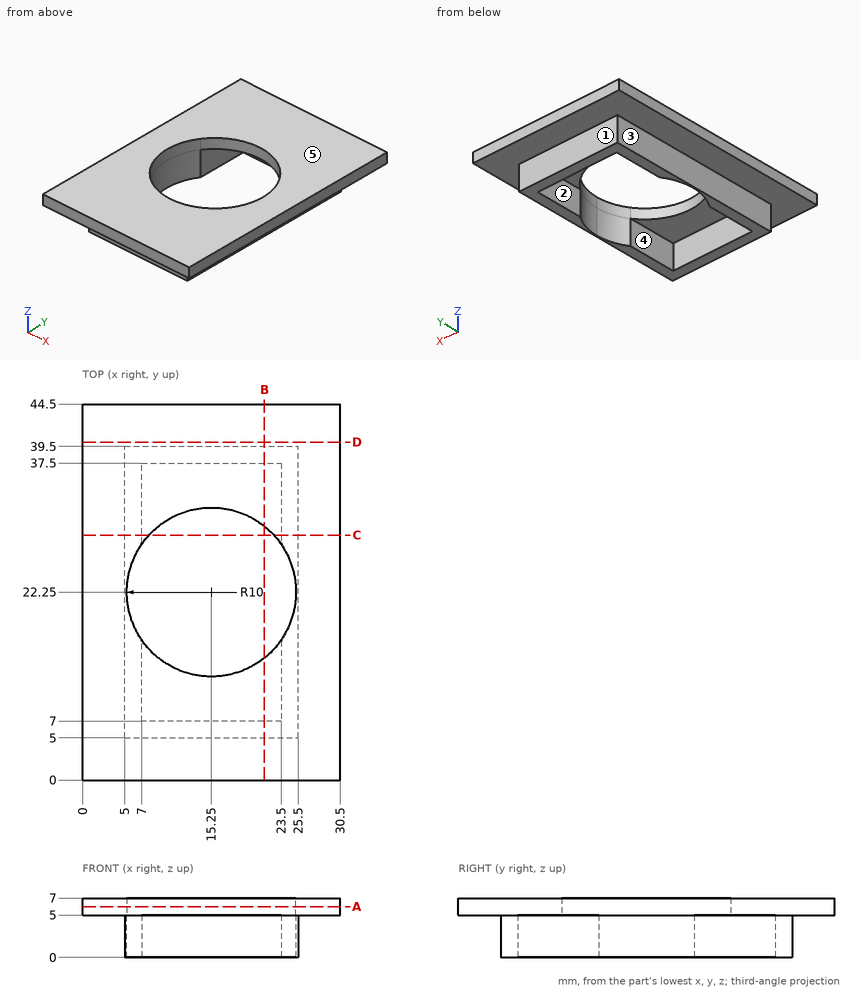
Here's the drawing with two shaded views (mm, measured from the low corner). I have some questions. A direction names the side the tool comes from. Round coordinates to 2 decimals unless told otherwise and drop trailing zeros. Order: outer loops, then holes, each group sorted by start corner. A loop starts at its lowest first (then second) coordinate and runs counter-clockwise, first axis right, second up. Notation, with made-up numbers: M 63.25,14 L 110.25,14 A35 ccw 110.25,47 Z; hole C 38.5,26 d9. An arc over 180 degrees is marked long. Answer in a Markdown table with one row per item.
Item 1: Imagine slicing it at A-A, the plane z = 6. Write out the boundary of the cut face in (x, y).
A:
| item | result |
|---|---|
| outline | M 0,0 L 30.5,0 L 30.5,44.5 L 0,44.5 Z; hole C 15.25,22.25 d20 |
Item 2: Imagine slicing it at D-D, the plane y = 40. Write out the boundary of the cut face in (x, z), and give its area (3 significant figures).
A:
| item | result |
|---|---|
| outline | M 0,5 L 30.5,5 L 30.5,7 L 0,7 Z |
| area | 61.0 mm2 |
Item 3: I'm going to push flat-ended pins straight in: pin 1 (10.5 mm diameter, centred on x = 17, y = 13.5, fed in from -Z); pin 2 (1.5 mm diameter, centred on x = 12.5, z = 2.5, fed in from -Y); pin 3 (1.5 mm diameter, centred on y = 11.5, z = 2, fed in from +X); pin 4 (4 mm diameter, centred on x = 23.5, z = 4.5, fed in from -Y). Where does each tip first touch, or does it pass through?
A:
| item | result |
|---|---|
| pin 1 | stops at z = 5 |
| pin 2 | stops at y = 5 |
| pin 3 | stops at x = 25.5 |
| pin 4 | stops at y = 0 |
Item 4: Imagine slicing it at B-B, the plane x = 21.5. Write out the boundary of the cut face in (y, z), and give its area (3 significant figures).
A:
| item | result |
|---|---|
| outline | M 0,5 L 5,5 L 5,0 L 7,0 L 7,5 L 14.44,5 L 14.44,7 L 0,7 Z; M 30.06,5 L 37.5,5 L 37.5,0 L 39.5,0 L 39.5,5 L 44.5,5 L 44.5,7 L 30.06,7 Z |
| area | 77.8 mm2 |
Item 5: If I drill on L1, parallel to X at y = 35, z = 1.5; L2, parallel to Y at x = 10.5, z = 0.75; L3, parallel to Y at x = 15.5, z = 5.25, over which ranges is the centre line in solid material (lowest first)? Write a range as from..to.
A:
| item | result |
|---|---|
| L1 | x = 5..7, 23.5..25.5 |
| L2 | y = 5..7, 37.5..39.5 |
| L3 | y = 0..12.25, 32.25..44.5 |
Item 6: Thinking about a two-plate mould opening in X: for the marked faces 1, 2 and 3, which applies, +X half, -X half, draft (parallel to the pull), parting line (faces both ways), or undercut?
A:
| item | result |
|---|---|
| face 1 | draft |
| face 2 | undercut |
| face 3 | -X half |
Item 7: For the marked faces 4 and 5, which set-ups out of +Z, -Z, +X, -X, +Y, -Y let a thin tool reach every point of the face, with its end or its side?
A:
| item | result |
|---|---|
| face 4 | -Z |
| face 5 | +Z, +X, -X, +Y, -Y |
Item 8: Imagine slicing it at C-C, the plane y = 29. Write out the boundary of the cut face in (x, z).
A:
| item | result |
|---|---|
| outline | M 0,5 L 5,5 L 5,0 L 7,0 L 7,5 L 7.87,5 L 7.87,7 L 0,7 Z; M 22.63,5 L 23.5,5 L 23.5,0 L 25.5,0 L 25.5,5 L 30.5,5 L 30.5,7 L 22.63,7 Z |
